Work out the finished part from the listing and answer in its coordinate system (mm). Face numbers are marked on the shaded views. Round coordinates to 2 decimals unless told otherwise and drop trailing zeros. Write each loop counter-clockwise with the first axis right and the second up, starting at its lowest first coordinate (ties: lowest second). Pieces come first, ordered by that corner, then holes.
1. Straight lines are drawn through the part: probe 1 along X at (y, z) = (0, -3.3); probe 2 along Y at (x, z) = (0, 3.1). For each, find the intervals that lie inside material, in ascending order.
2. Find section C-C (z = 1.75). Count the separate pieces of the cut face and the enclosed holes in it, and give its area (3 significant figures).
3. Find section B-B (x = -4.25). Write down the section's boundary in (y, z), and give its area (3 significant figures).
4. Determine the mould class of the marked faces 1, 2 and 3 for opening direction X: pulls with the +X half, pulls with the -X half, needs draft (parallel to the pull), parting line crosses it, or undercut.
5. Find section A-A (x = 0). Write down the section's boundary in (y, z).
6. A flat-ended cylindrical pin translates along its axis: pin 1 Ø5 at (x, z) = (5.5, 3.5) entering from +Y. Find the tip coordinate at first contact, or state that the pin passes through.
```python
from build123d import *

# Parameters (mm, degrees)
F0_W      = 10
F0_H      = 10
F1_DEPTH  = 10
F3_R      = 2
F4_DEPTH  = 14.143136
F6_R      = 2
F7_DEPTH  = 14.143136
F8_R      = 0.5
F9_DEPTH  = 10.001
F10_R     = 0.5
F11_DEPTH = 10.001


with BuildPart() as f1:
    # F0 (on Right) → F1 (new body, symmetric)
    with BuildSketch(Plane.YZ):
        Rectangle(F0_W, F0_H)
    extrude(amount=F1_DEPTH, both=True)

    # F3 (on face) → F4 (cut, through all)
    with BuildSketch(Plane(origin=(0, -5, 5), x_dir=(1, 0, 0), z_dir=(0, -0.707107, 0.707107))):
        with Locations((-5, 0)):
            Circle(F3_R)
    extrude(amount=-F4_DEPTH, mode=Mode.SUBTRACT)

    # F6 (on face) → F7 (cut, through all)
    with BuildSketch(Plane(origin=(0, 5, 5), x_dir=(1, 0, 0), z_dir=(0, -0.707107, -0.707107))):
        with Locations((5, 0)):
            Circle(F6_R)
    extrude(amount=F7_DEPTH, mode=Mode.SUBTRACT)

    # F8 (on face) → F9 (cut, through all)
    with BuildSketch(Plane(origin=(0, 5, 0), x_dir=(-1, 0, 0), z_dir=(0, 1, 0))):
        Circle(F8_R)
    extrude(amount=-F9_DEPTH, mode=Mode.SUBTRACT)

    # F10 (on face) → F11 (cut, through all)
    with BuildSketch(Plane.XY.offset(5)):
        Circle(F10_R)
    extrude(amount=-F11_DEPTH, mode=Mode.SUBTRACT)


solid = f1.part
```
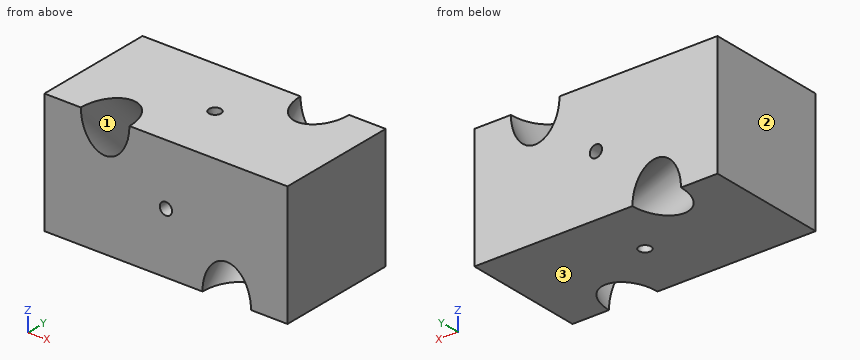
Worked answers:
1. probe 1: x = -10 to -0.5, 0.5 to 10
1. probe 2: y = -5 to -0.5, 0.5 to 5
2. separate pieces: 1
2. enclosed holes: 3
2. area: 164 mm2
3. outline: (-5, -5) - (2.38, -5) - (-5, 2.38) - close; (-2.38, 5) - (5, -2.38) - (5, 5) - close
3. area: 54.4 mm2
4. face 1: undercut
4. face 2: pulls with the -X half
4. face 3: needs draft
5. outline: (-5, -5) - (-0.5, -5) - (-0.5, -0.5) - (-5, -0.5) - close; (-5, 0.5) - (-0.5, 0.5) - (-0.5, 5) - (-5, 5) - close; (0.5, -5) - (5, -5) - (5, -0.5) - (0.5, -0.5) - close; (0.5, 0.5) - (5, 0.5) - (5, 5) - (0.5, 5) - close
6. pin 1: stops at y = 5
